For this review, take the finished solid that the model builds, in its own axes (mm). A direction names the side the tool comes from. Coordinates: 2 decimals unless noted, no trailing zeros. Write each loop counter-clockwise with the first axis right and the second up, starting at its lowest first coordinate (ties: lowest second). Pieces come first, ordered by that corner, then holes. Notation, with made-up numbers: (-27, -35) -> (27, -35) arc R18 cw to (27, -30) -> close; hole circle Ø1 at (89, -0.5). An arc over 180 degrees is marked (long way). One line per item, written item: value. Start each with the question number.
1) Add section A-A (z = -78). State the section outline as (x, y) points, and give its area (3 significant figures).
2) For probe 1 along Z at (x, y) = (-190, 3.3); probe 2 along X at (y, z) = (1, -90); probe 3 along Y at (x, z) = (-162.5, -60), list the stretches that pass through material, from the lowest coordinate up. Write a range as from..to.
3) Machinability: for faces 1 (the flat face through (-99, 25, -30)), 2 (the flat face through (-99, 0, -49)), which of the approach directions +Z, -Z, +X, -X, +Y, -Y give a long, thin tool a straight path to every point of the face, cutting with its end or side? Answer none if there is none.
4) Add section D-D (y = 34.5). State the section outline as (x, z) points.
5) Add section C-C (y = 8). State the section outline as (x, z) points.
6) For pin 1 Ø10 at (x, y) = (-131, 28) entering from +Z; pin 2 Ø2.5 at (x, z) = (-190, -10) entering from -Y; pin 3 Ø8 at (x, y) = (-177, 37) entering from -Z, all flat-tipped, find the tip position at first contact; note any pin that passes through.
7) Add section B-B (x = -157.5). State the section outline as (y, z) points.
Autodesk Inventor part; units mm, degrees
ref_plane "YZ Plane" through (0, 0, 0) normal (1, 0, 0) x (0, 1, 0)
ref_plane "XZ Plane" through (0, 0, 0) normal (0, 1, 0) x (-1, 0, 0)
ref_plane "XY Plane" through (0, 0, 0) normal (0, 0, 1) x (1, 0, 0)
sketch "Sketch1" plane through (0, 0, 0) normal (1, 0, 0) x (0, 1, 0)
  line L0 (0, 0) -> (0, -100)
  line L1 (0, -100) -> (50, -100)
  line L2 (50, -100) -> (50, -29.2097)
  arc A0 (50, -29.2097) -> (0, 0) centre (2.9206, -52.3995) ccw
  dimension "d0" = 100
  dimension "d1" = 50
extrude "Extrusion1" add sketch "Sketch1" against normal blind 200
sketch "Sketch4" plane through (0, 0, -100) normal (0, 0, -1) x (-1, 0, 0)
  line L0 (5, 45) -> (5, 5)
  line L1 (5, 5) -> (195, 5)
  line L2 (195, 5) -> (195, 45)
  line L3 (195, 45) -> (5, 45)
  line L4 (0, 50) -> (200, 50)
  line L5 (0, 0) -> (0, 50)
  line L6 (200, 50) -> (200, 0)
  line L7 (0, 0) -> (200, 0)
  dimension "d5" = 5
  dimension "d6" = 5
  dimension "d7" = 5
  dimension "d8" = 5
extrude "Extrusion2" cut sketch "Sketch4" against normal blind 70 contours L3 L2 L1 L0
sketch "Sketch5" plane through (0, 0, -100) normal (0, -1, 0) x (1, 0, 0)
  circle A0 centre (-10, 90) radius 1.5
  circle A1 centre (-10, 10) radius 1.5
  circle A2 centre (-190, 90) radius 1.5
  circle A3 centre (-190, 10) radius 1.5
  line L0 (0, 100) -> (-200, 100)
  line L1 (0, 0) -> (-200, 0)
  line L2 (0, 100) -> (0, 0)
  line L3 (-200, 0) -> (-200, 100)
  point P0 (-195, 0)
  dimension "d11" = 3
  dimension "d12" = 3
  dimension "d13" = 3
  dimension "d14" = 3
  dimension "d15" = 10
  dimension "d16" = 10
  dimension "d17" = 10
  dimension "d18" = 10
  dimension "d19" = 10
  dimension "d20" = 10
  dimension "d22" = 10
  dimension "d23" = 10
extrude "Extrusion3" cut sketch "Sketch5" against normal blind 10 contours A0 | A1 | A2 | A3
equation "\"d1\" = 0.5 * d0"
equation "\"d16\" = d15"
equation "\"d18\" = d17"
equation "\"d19\" = d17"
equation "\"d20\" = d15"
equation "\"d22\" = d17"
equation "\"d23\" = d15"
properties part number "Container"
Numbers:
1. outline: (-200, 0) -> (0, 0) -> (0, 50) -> (-200, 50) -> close; hole (-195, 5) -> (-5, 5) -> (-5, 45) -> (-195, 45) -> close
1. area: 2,400 mm²
2. probe 1: -100..-91.5, -88.5..-11.5, -8.5..0.08
2. probe 2: -200..-191.5, -188.5..-11.5, -8.5..0
2. probe 3: 0..5, 45..50
3. face 1: -Z
3. face 2: +Z, -Z, +X, -X, -Y
4. outline: (-200, -100) -> (-195, -100) -> (-195, -30) -> (-5, -30) -> (-5, -100) -> (0, -100) -> (0, -10.48) -> (-200, -10.48) -> close
5. outline: (-200, -100) -> (-195, -100) -> (-195, -30) -> (-5, -30) -> (-5, -100) -> (0, -100) -> (0, -0.17) -> (-200, -0.17) -> close; hole circle Ø3 at (-190, -10); hole circle Ø3 at (-10, -10)
6. pin 1: z = -3.91
6. pin 2: y = 10
6. pin 3: z = -30
7. outline: (0, -100) -> (5, -100) -> (5, -30) -> (45, -30) -> (45, -100) -> (50, -100) -> (50, -29.21) arc R52.48 ccw to (0, 0) -> close
